from build123d import *

# Parameters (mm, degrees)
CHAMFER1_SIZE = 1.5


with BuildPart() as part:
    # Sketch2 → Revolve1 (revolve)
    with BuildSketch(Plane.XY):
        with BuildLine():
            Line((0, 0), (26.67, 0))
            Line((26.67, 0), (26.67, 1.27))
            Line((26.67, 1.27), (24.13, 3.81))
            ThreePointArc((24.13, 3.81), (9.893843865, 5.312197185), (3.175, 17.952682737))
            Line((3.175, 17.952682737), (3.175, 85.55))
            Line((3.175, 85.55), (0, 85.55))
            Line((0, 85.55), (0, 0))
        make_face()
    revolve(axis=Axis((0, 85.55, 0), (0, -1, 0)))

    # Chamfer1
    chamfer1_edges = [part.edges().sort_by_distance(p)[0] for p in [
        (-3.175, 85.55, 0),
    ]]
    chamfer(chamfer1_edges, length=CHAMFER1_SIZE)


solid = part.part
Can you work these out from the model? Positions are in its coordinate system, mm. A direction names the side the tool comes from. Round coordinates to 2 decimals unless told otherwise and drop trailing zeros. Loops run counter-clockwise (first coordinate to the right, second up) from the corner with the lowest first, then second, coordinate; pieces in that order, holes last. Notation, with made-up numbers: (46, -2) - (69, -2) arc R19 cw to (69, 8) - close; hole circle Ø9 at (61, 60.25). An arc over 180 degrees is marked (long way). Use CSV: the item, a comma, the result in double quotes. Start each with the question number.
1) For faces 1 (the flat face through (0, 85.55, 0)), 2 (the cylindrical face through (-0.69, 51.46, -3.1)), which set-ups out of +Z, -Z, +X, -X, +Y, -Y let a thin tool reach every point of the face, with its end or its side?
2) If we section it at A-A on z = 0: Write out the boundary of the cut face in (x, y) (3 decimals), plus the area to 3 significant figures.
3) If we section it at B-B on x = 0: Write out the boundary of the cut face in (y, z) (3 decimals), plus the area to 3 significant figures.
4) For pin 1 Ø12 at (x, z) = (-15.5, -5.5) entering from -Y; pin 2 Ø1.5 at (y, z) = (35, 0.5) entering from +X (3 decimals); pin 3 Ø3 at (x, z) = (-20.5, 3) entering from +Y; pin 4 Ø10 at (x, z) = (-12, -8.5) entering from +Y, each with a flat end and sliding along its axis, tell me the tip position at first contact or that it passes through.
5) If we section it at C-C on y = 24: Write out the boundary of the cut face in (x, z) (3 decimals), plus the area to 3 significant figures.
6) If we section it at D-D on y = 8: Write out the boundary of the cut face in (x, z), plus the area to 3 significant figures.
7) Please list where these lines run through material, in increasing order: probe 1 along Z at (x, y) = (0, 61.5) (3 decimals); probe 2 along Y at (x, z) = (-16.5, 8.5); probe 3 along Z at (x, y) = (0.5, 55.5). Write a range as [from, to].
Geometry results:
1,face 1,"+Z, -Z, +X, -X, +Y"
1,face 2,"+Y"
2,outline,"(-26.67, 0) - (26.67, 0) - (26.67, 1.27) - (24.13, 3.81) arc R15.25 cw to (3.175, 17.953) - (3.175, 84.05) - (1.675, 85.55) - (-1.675, 85.55) - (-3.175, 84.05) - (-3.175, 17.953) arc R15.25 cw to (-24.13, 3.81) - (-26.67, 1.27) - close"
2,area,"771 mm2"
3,outline,"(0, -26.67) - (1.27, -26.67) - (3.81, -24.13) arc R15.25 cw to (17.953, -3.175) - (84.05, -3.175) - (85.55, -1.675) - (85.55, 1.675) - (84.05, 3.175) - (17.953, 3.175) arc R15.25 cw to (3.81, 24.13) - (1.27, 26.67) - (0, 26.67) - close"
3,area,"771 mm2"
4,pin 1,"stops at y = 0"
4,pin 2,"stops at x = 3.175"
4,pin 3,"stops at y = 3.18"
4,pin 4,"stops at y = 5.44"
5,outline,"circle Ø6.35 at (0, 0)"
5,area,"31.7 mm2"
6,outline,"circle Ø13.74 at (0, 0)"
6,area,"148 mm2"
7,probe 1,"z = [-3.175, 3.175]"
7,probe 2,"y = [0, 2.7]"
7,probe 3,"z = [-3.14, 3.14]"
